```python
from build123d import *

# Parameters (mm, degrees)
CROQUIS1_W              = 65
CROQUIS1_H              = 25
SALIENTE_EXTRUIR1_DEPTH = 10
CROQUIS2_W              = 60
CROQUIS2_H              = 22.4
CORTAR_EXTRUIR1_DEPTH   = 8.5
SKETCH3_R               = 3
BOSS_EXTRUDE3_DEPTH     = 3
SKETCH4_R               = 1.15
BOSS_EXTRUDE4_DEPTH     = 5.3
CORTAR_EXTRUIR3_REACH   = 68.942
CROQUIS5_W              = 6
CROQUIS5_H              = 8
CROQUIS12_W             = 33
CROQUIS12_H             = 16
SALIENTE_EXTRUIR7_DEPTH = 10
CROQUIS13_W             = 28
CROQUIS13_H             = 16
CORTAR_EXTRUIR6_DEPTH   = 8.5
CROQUIS14_R             = 2
SALIENTE_EXTRUIR8_DEPTH = 3
CROQUIS15_R             = 1.4
SALIENTE_EXTRUIR9_DEPTH = 3


with BuildPart() as part:
    # Croquis1 → Saliente-Extruir1 (new body)
    with BuildSketch(Plane(origin=(0, 0, 0), x_dir=(1, 0, 0), z_dir=(0, 1, 0))):
        Rectangle(CROQUIS1_W, CROQUIS1_H)
    extrude(amount=SALIENTE_EXTRUIR1_DEPTH)

    # Croquis2 → Cortar-Extruir1 (cut)
    with BuildSketch(Plane(origin=(0, 10, 0), x_dir=(1, 0, 0), z_dir=(0, 1, 0))):
        Rectangle(CROQUIS2_W, CROQUIS2_H)
    extrude(amount=-CORTAR_EXTRUIR1_DEPTH, mode=Mode.SUBTRACT)

    # Sketch3 → Boss-Extrude3 (add)
    with BuildSketch(Plane(origin=(0, 1.5, 0), x_dir=(1, 0, 0), z_dir=(0, 1, 0))):
        with Locations(Location((-24.05, 0, 0), (0, 0, 270))):
            Circle(SKETCH3_R)
        with Locations(Location((22.55, 7.55, 0), (0, 0, 270))):
            Circle(SKETCH3_R)
        with Locations(Location((22.55, -7.55, 0), (0, 0, 90))):
            Circle(SKETCH3_R)
    extrude(amount=BOSS_EXTRUDE3_DEPTH)

    # Sketch4 → Boss-Extrude4 (add)
    with BuildSketch(Plane(origin=(0, 4.5, 0), x_dir=(1, 0, 0), z_dir=(0, 1, 0))):
        with Locations(Location((-24.05, 0, 0), (0, 0, 270))):
            Circle(SKETCH4_R)
        with Locations(Location((22.55, 7.55, 0), (0, 0, 270))):
            Circle(SKETCH4_R)
        with Locations(Location((22.55, -7.55, 0), (0, 0, 270))):
            Circle(SKETCH4_R)
    extrude(amount=BOSS_EXTRUDE4_DEPTH)

    # Croquis5 → Cortar-Extruir3 (cut, up to next)
    with BuildSketch(Plane(origin=(32.5, 0, 0), x_dir=(0, 0, -1), z_dir=(1, 0, 0)), mode=Mode.PRIVATE) as cortar_extruir3_sk1:
        with Locations((0, 6)):
            Rectangle(CROQUIS5_W, CROQUIS5_H)
    cortar_extruir3_tool1 = extrude(cortar_extruir3_sk1.sketch, amount=-CORTAR_EXTRUIR3_REACH, mode=Mode.PRIVATE) & part.part
    add(cortar_extruir3_tool1.solids().sort_by_distance((32.5, 6, 0))[0], mode=Mode.SUBTRACT)

    # Croquis12 → Saliente-Extruir7 (add)
    with BuildSketch(Plane(origin=(0, 0, 0), x_dir=(1, 0, 0), z_dir=(0, 1, 0))):
        with Locations((0, -20.5)):
            Rectangle(CROQUIS12_W, CROQUIS12_H)
    extrude(amount=SALIENTE_EXTRUIR7_DEPTH)

    # Croquis13 → Cortar-Extruir6 (cut)
    with BuildSketch(Plane(origin=(0, 10, 0), x_dir=(1, 0, 0), z_dir=(0, 1, 0))):
        with Locations((0, -19.2)):
            Rectangle(CROQUIS13_W, CROQUIS13_H)
    extrude(amount=-CORTAR_EXTRUIR6_DEPTH, mode=Mode.SUBTRACT)

    # Croquis14 → Saliente-Extruir8 (add)
    with BuildSketch(Plane(origin=(0, 1.5, 0), x_dir=(1, 0, 0), z_dir=(0, 1, 0))):
        with Locations(Location((8, -14.2, 0), (0, 0, 270))):
            Circle(CROQUIS14_R)
        with Locations(Location((8, -24.2, 0), (0, 0, 90))):
            Circle(CROQUIS14_R)
        with Locations(Location((-8, -24.2, 0), (0, 0, 270))):
            Circle(CROQUIS14_R)
        with Locations(Location((-8, -14.2, 0), (0, 0, 90))):
            Circle(CROQUIS14_R)
    extrude(amount=SALIENTE_EXTRUIR8_DEPTH)

    # Croquis15 → Saliente-Extruir9 (add)
    with BuildSketch(Plane(origin=(0, 4.5, 0), x_dir=(1, 0, 0), z_dir=(0, 1, 0))):
        with Locations(Location((8, -14.2, 0), (0, 0, 270))):
            Circle(CROQUIS15_R)
    extrude(amount=SALIENTE_EXTRUIR9_DEPTH)


solid = part.part
```
Work out the finished part from the listing and answer in its coordinate system (mm). A direction names the side the tool comes from. Round coordinates to 2 decimals unless told otherwise and drop trailing zeros. Loops run counter-clockwise (first coordinate to the right, second up) from the corner with the lowest first, then second, coordinate; pieces in that order, holes last.
(1) The part is cut by section D-D, the plane z = 19. Give the vertices of the cut face in (x, y), and give its area (3 significant figures).
Computed values:
outline: (-16.5, 0) - (16.5, 0) - (16.5, 10) - (14, 10) - (14, 1.5) - (-14, 1.5) - (-14, 10) - (-16.5, 10) - close
area: 92.0 mm2
(2) The part is cut by section B-B, the plane z = 0. Give the vertices of the cut face in (x, y).
Computed values:
outline: (-32.5, 0) - (32.5, 0) - (32.5, 2) - (30, 2) - (30, 1.5) - (-21.05, 1.5) - (-21.05, 4.5) - (-22.9, 4.5) - (-22.9, 9.8) - (-25.2, 9.8) - (-25.2, 4.5) - (-27.05, 4.5) - (-27.05, 1.5) - (-30, 1.5) - (-30, 10) - (-32.5, 10) - close
(3) The mould has two halves that part along Z. Classify faces 5 (the flat face through (31, 6, 3)), 6 (the flat face through (0, 5, 28.5)), 7 (the flat face through (-15, 10, 14)): pulls with the +Z half, pulls with the -Z half, needs draft (parallel to the pull), parting line crosses it, or undercut.
Computed values:
face 5: undercut
face 6: pulls with the +Z half
face 7: needs draft
(4) The part is cut by section C-C, the plane x = 22.55. Give the vertices of the cut face in (y, z).
Computed values:
outline: (0, -12.5) - (10, -12.5) - (10, -11.2) - (1.5, -11.2) - (1.5, -10.55) - (4.5, -10.55) - (4.5, -8.7) - (9.8, -8.7) - (9.8, -6.4) - (4.5, -6.4) - (4.5, -4.55) - (1.5, -4.55) - (1.5, 4.55) - (4.5, 4.55) - (4.5, 6.4) - (9.8, 6.4) - (9.8, 8.7) - (4.5, 8.7) - (4.5, 10.55) - (1.5, 10.55) - (1.5, 11.2) - (10, 11.2) - (10, 12.5) - (0, 12.5) - close
(5) For faces 1 (the flat face through (31, 6, -3)), 2 (the flat face through (-25, 5, 12.5)), 3 (the flat face through (21, 4.5, -8)), 4 (the flat face through (0, 0, 3)), determine the directions among +Z, -Z, +X, -X, +Y, -Y from which every point of the face is accessible in a straight line to the end or side of a thin tool.
Computed values:
face 1: +X, +Y
face 2: +Z, -X, +Y, -Y
face 3: +Y
face 4: +Z, -Z, +X, -X, -Y
(6) The part is cut by section A-A, the plane y = 9. Give the vertices of the cut face in (x, z).
Computed values:
outline: (-32.5, -12.5) - (32.5, -12.5) - (32.5, -3) - (30, -3) - (30, -11.2) - (-30, -11.2) - (-30, 11.2) - (-14, 11.2) - (-14, 27.2) - (14, 27.2) - (14, 11.2) - (30, 11.2) - (30, 3) - (32.5, 3) - (32.5, 12.5) - (16.5, 12.5) - (16.5, 28.5) - (-16.5, 28.5) - (-16.5, 12.5) - (-32.5, 12.5) - close; circle Ø2.3 at (-24.05, 0); circle Ø2.3 at (22.55, -7.55); circle Ø2.3 at (22.55, 7.55)
(7) Find the intervals of material crossed by L1, parallel to X at y = 7.75, z = -4; L2, parallel to Z at x = 24, y = 8.5; L3, parallel to X at y = 5, z = 16.5, in increasing order.
Computed values:
L1: x = -32.5 to -30, 30 to 32.5
L2: z = -12.5 to -11.2, 11.2 to 12.5
L3: x = -16.5 to -14, 14 to 16.5
(8) Each of these flat-tipped pins is pushed along its axis until it touches: P1, Ø3, axis at x = -7, z = 8.5, coming from the +Y side; P2, Ø3, axis at x = 31.5, z = 0.5, coming from the +Y side; P3, Ø1, axis at y = 8.5, z = 2, coming from the +X side. Where does it stop, or does it pass through?
Computed values:
P1: stops at y = 1.5
P2: stops at y = 2
P3: stops at x = -30
